Input: part model. Units: mm. Frame: model coordinates. Face numbers are marked on the shaded views. A direction names the side the tool comes from. Coordinates: 2 decimals unless noted, no trailing zeros. Order: outer loops, then holes, each group sorted by start corner. A loop starts at its lowest first (then second) coordinate and runs counter-clockwise, first axis right, second up. Notation, with made-up numbers: (47.5, 14) - (97.5, 14) arc R24 cw to (97.5, 53) - close; hole circle Ø6 at (26.25, 80). An arc over 180 degrees is marked (long way). Use a Markdown table: item, result. Add a question column.
from build123d import *

# Parameters (mm, degrees)
SZKIC1_R                    = 4.5
SZKIC1_R_2                  = 3
DODANIE_WYCI_GNI_CIE1_DEPTH = 24
WYTNIJ_WYCI_GNI_CIE1_DEPTH  = 3


with BuildPart() as part:
    # Szkic1 → Dodanie-wyciągnięcie1 (new body)
    with BuildSketch(Plane(origin=(0, 0, 0), x_dir=(0, 0, -1), z_dir=(1, 0, 0))):
        Circle(SZKIC1_R)
        Circle(SZKIC1_R_2, mode=Mode.SUBTRACT)
    extrude(amount=DODANIE_WYCI_GNI_CIE1_DEPTH)

    # Szkic2 → Wytnij-wyciągnięcie1 (cut)
    with BuildSketch(Plane(origin=(24, 0, 0), x_dir=(0, 0, -1), z_dir=(1, 0, 0))):
        Polygon((4.041451884, 0), (2.020725942, 3.5), (-2.020725942, 3.5), (-4.041451884, 0), (-2.020725942, -3.5), (2.020725942, -3.5), align=None)
    extrude(amount=-WYTNIJ_WYCI_GNI_CIE1_DEPTH, mode=Mode.SUBTRACT)


solid = part.part
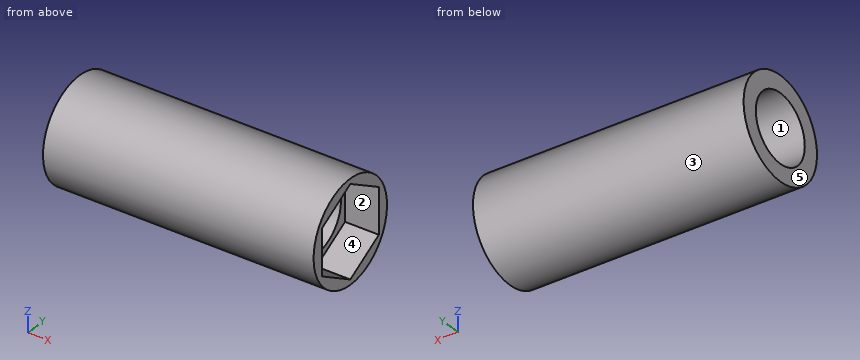
1) Cut plane A-A (z = -1.5). Return the cut outline in (x, y), and give its area (3 significant figures).
2) Cut plane B-B (y = -2). Return the cut outline in (x, z).
3) Contact query for flat-ended pins moving along their axis: P1, Ø4, axis at y = -1.5, z = -3.5, coming from the -X side; P2, Ø1, axis at x = 18.5, y = -1, coming from the -Z side. Output: stop coordinate, or through.
4) Cut plane D-D (z = 3.25). Return the cut outline in (x, y), and give its area (3 significant figures).
5) Cut plane C-C (x = 7.75). Return the cut outline in (y, z), and give its area (3 significant figures).
6) Material intervals for L1, parallel to Y at x = 7.25, z = 0; L2, parallel to Y at x = 8.25, z = -1.5; L3, parallel to Z at x = 7.75, y = -1, sorted ascending.
7) Pull-direction query (Z, two-part tool) for the marked faces 3, 4 and 5; classes: pulls with the +Z half, pulls with the -Z half, needs draft (parallel to the pull), parting line crosses it, or undercut.
8) Reachability of the marked faces 1 and 2 from +Z, -Z, +X, -X, +Y, -Y: full face, straight path, thin tool, end or side. Return the list, or none.
Computed:
| question | item | result |
|---|---|---|
| 1 | outline | (0, -4.24) - (24, -4.24) - (24, -3.5) - (21, -3.5) - (21, -2.6) - (0, -2.6) - close; (0, 2.6) - (21, 2.6) - (21, 3.5) - (24, 3.5) - (24, 4.24) - (0, 4.24) - close |
| 1 | area | 73.5 mm2 |
| 2 | outline | (0, -4.03) - (24, -4.03) - (24, -2.89) - (21, -2.89) - (21, -2.24) - (0, -2.24) - close; (0, 2.24) - (21, 2.24) - (21, 2.89) - (24, 2.89) - (24, 4.03) - (0, 4.03) - close |
| 3 | P1 | stops at x = 0 |
| 3 | P2 | stops at z = -4.47 |
| 4 | outline | (0, -3.11) - (24, -3.11) - (24, -1.37) - (21, -1.37) - (21, 1.37) - (24, 1.37) - (24, 3.11) - (0, 3.11) - close |
| 4 | area | 141 mm2 |
| 5 | outline | circle Ø9 at (0, 0); hole circle Ø6 at (0, 0) |
| 5 | area | 35.3 mm2 |
| 6 | L1 | y = -4.5 to -3, 3 to 4.5 |
| 6 | L2 | y = -4.24 to -2.6, 2.6 to 4.24 |
| 6 | L3 | z = -4.39 to -2.83, 2.83 to 4.39 |
| 7 | face 3 | parting line crosses it |
| 7 | face 4 | undercut |
| 7 | face 5 | needs draft |
| 8 | face 1 | +X, -X |
| 8 | face 2 | +X |
